from build123d import *

# Parameters (mm, degrees)
SKETCH1_R           = 79.375
SKETCH1_R_2         = 1.4224
BOSS_EXTRUDE1_DEPTH = 3.048


with BuildPart() as part:
    # Sketch1 → Boss-Extrude1 (new body)
    with BuildSketch(Plane(origin=(0, 0, 0), x_dir=(1, 0, 0), z_dir=(0, 1, 0))):
        Circle(SKETCH1_R)
        with Locations((0, 73.025)):
            Circle(SKETCH1_R_2, mode=Mode.SUBTRACT)
        with Locations((27.945457648, 67.466302862)):
            Circle(SKETCH1_R_2, mode=Mode.SUBTRACT)
        with Locations((51.636472696, 51.636472696)):
            Circle(SKETCH1_R_2, mode=Mode.SUBTRACT)
        with Locations((67.466302862, 27.945457648)):
            Circle(SKETCH1_R_2, mode=Mode.SUBTRACT)
        with Locations((73.025, 0)):
            Circle(SKETCH1_R_2, mode=Mode.SUBTRACT)
        with Locations((67.466302862, -27.945457648)):
            Circle(SKETCH1_R_2, mode=Mode.SUBTRACT)
        with Locations((51.636472696, -51.636472696)):
            Circle(SKETCH1_R_2, mode=Mode.SUBTRACT)
        with Locations((27.945457648, -67.466302862)):
            Circle(SKETCH1_R_2, mode=Mode.SUBTRACT)
        with Locations((0, -73.025)):
            Circle(SKETCH1_R_2, mode=Mode.SUBTRACT)
        with Locations((-27.945457648, -67.466302862)):
            Circle(SKETCH1_R_2, mode=Mode.SUBTRACT)
        with Locations((-51.636472696, -51.636472696)):
            Circle(SKETCH1_R_2, mode=Mode.SUBTRACT)
        with Locations((-67.466302862, -27.945457648)):
            Circle(SKETCH1_R_2, mode=Mode.SUBTRACT)
        with Locations((-73.025, 0)):
            Circle(SKETCH1_R_2, mode=Mode.SUBTRACT)
        with Locations((-67.466302862, 27.945457648)):
            Circle(SKETCH1_R_2, mode=Mode.SUBTRACT)
        with Locations((-51.636472696, 51.636472696)):
            Circle(SKETCH1_R_2, mode=Mode.SUBTRACT)
        with Locations((-27.945457648, 67.466302862)):
            Circle(SKETCH1_R_2, mode=Mode.SUBTRACT)
    extrude(amount=BOSS_EXTRUDE1_DEPTH)


solid = part.part
Here's how the part is built. I have some questions about the finished solid (model axes, mm). Give positions to 0.01 mm unless a question says otherwise; leave off trailing zeros. Loops run counter-clockwise (first coordinate to the right, second up) from the corner with the lowest first, then second, coordinate; pieces in that order, holes last. Notation, with made-up numbers: (51.5, 19.25) -> (66.5, 19.25) arc R10 cw to (66.5, 23.25) -> close; hole circle Ø3 at (-21, -38). An arc over 180 degrees is marked (long way). Answer as a JSON object with one key per item and string values. Group by question number.
Item 1: Imagine slicing it at A-A on y = 2. Give the number of separate pieces and of enclosed holes in the cut face, then the cut area to 3 significant figures.
Item 2: Will these pins go through, and if not, where does the flat tip stop? pin 1 (2.5 mm diameter, centred on x = -51.64, z = 51.64, fed in from +Y); pin 2 (2 mm diameter, centred on x = 62, z = -1, fed in from -Y).
Item 3: Imagine slicing it at C-C on z = -15. Write out the boundary of the cut face in (x, y), then the cut area to 3 significant figures.
Item 4: I need wall thicknesses on L1, parallel to X at y = 1.65, z = 0 (3 decimals); L2, parallel to X at y = 1.95, z = -27.5; L3, parallel to X at y = 1.45, z = 3.5. Which ranges of each line are inside material? Lowest first, please.
Item 5: Imagine slicing it at B-B on z = 18. Write out the boundary of the cut face in (x, y), then the cut area to 3 significant figures.
Answer list:
{
 "1": {"separate pieces": "1", "enclosed holes": "16", "area": "19,700 mm2"},
 "2": {"pin 1": "passes through", "pin 2": "stops at y = 0"},
 "3": {"outline": "(-77.94, 0) -> (77.94, 0) -> (77.94, 3.05) -> (-77.94, 3.05) -> close", "area": "475 mm2"},
 "4": {"L1": "x = -79.375 to -74.447, -71.603 to 71.603, 74.447 to 79.375", "L2": "x = -74.46 to -68.82, -66.12 to 66.12, 68.82 to 74.46", "L3": "x = -79.3 to 79.3"},
 "5": {"outline": "(-77.31, 0) -> (77.31, 0) -> (77.31, 3.05) -> (-77.31, 3.05) -> close", "area": "471 mm2"}
}
